Read the model definition and answer for the solid it produces. Units are mm, in the model's axes. Face numbers are marked on the shaded views. A direction names the side the tool comes from. Round coordinates to 2 decimals unless told otherwise and drop trailing zeros. Loops run counter-clockwise (first coordinate to the right, second up) from the corner with the lowest first, then second, coordinate; pieces in that order, holes last. Notation, with made-up numbers: M 57.25,77 L 83.25,77 A23 cw 83.25,105 Z; hole C 42.5,32.25 d1. An arc over 180 degrees is marked long. Write each question's results on one line, items separated by ' | '.
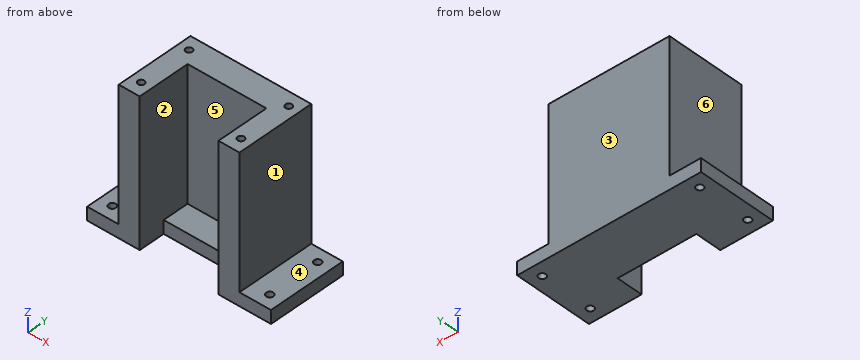
```python
from build123d import *

# Parameters (mm, degrees)
SKETCH_1_R               = 1.35
EXTRUDE_1_DEPTH          = 5
EXTRUDE_2_DEPTH          = 50
SKETCH_3_R               = 1.25
CUT_EXTRUDE_1_DEPTH      = 10
MIRROR_2_COPY_1_SKETCH_R = 1.25
MIRROR_2_COPY_1_DEPTH    = 10


with BuildPart() as part:
    # Sketch 1 → Extrude 1 (new body)
    with BuildSketch(Plane.XY):
        Polygon((20, 0), (20, 10), (50, 10), (50, 0), (70, 0), (70, 30), (0, 30), (0, 0), align=None)
        with Locations((5, 25)):
            Circle(SKETCH_1_R, mode=Mode.SUBTRACT)
        with Locations((5, 5)):
            Circle(SKETCH_1_R, mode=Mode.SUBTRACT)
        with Locations((65, 25)):
            Circle(SKETCH_1_R, mode=Mode.SUBTRACT)
        with Locations((65, 5)):
            Circle(SKETCH_1_R, mode=Mode.SUBTRACT)
    extrude(amount=EXTRUDE_1_DEPTH)

    # Sketch 2 → Extrude 2 (add)
    with BuildSketch(Plane.XY.offset(5)):
        Polygon((20, 20), (20, 0), (12, 0), (12, 30), (58, 30), (58, 0), (50, 0), (50, 20), align=None)
    extrude(amount=EXTRUDE_2_DEPTH)

    # Sketch 3 → Cut-Extrude 1 (cut)
    with BuildSketch(Plane.XY.offset(55)):
        with Locations((16, 25)):
            Circle(SKETCH_3_R)
    cut_extrude_1 = extrude(amount=-CUT_EXTRUDE_1_DEPTH, mode=Mode.SUBTRACT)

    # Mirror 1: Cut-Extrude 1 across plane
    add(cut_extrude_1.mirror(Plane(origin=(35, 0, 0), x_dir=(0, 0, 1), z_dir=(1, 0, 0))), mode=Mode.SUBTRACT)

    # Mirror 2: Cut-Extrude 1 across plane
    add(cut_extrude_1.mirror(Plane.ZX.offset(15)), mode=Mode.SUBTRACT)

    # Mirror 2 copy 1 sketch → Mirror 2 copy 1 (cut)
    with BuildSketch(Plane(origin=(70, 30, 55), x_dir=(-1, 0, 0), z_dir=(0, 0, 1))):
        with Locations((16, 25)):
            Circle(MIRROR_2_COPY_1_SKETCH_R)
    extrude(amount=-MIRROR_2_COPY_1_DEPTH, mode=Mode.SUBTRACT)


solid = part.part
```
1. Which of the six approach directions +Z, -Z, +X, -X, +Y, -Y give full straight-line access (tool end or side, diameter ignored) to the marked faces 4, 5 and 6?
Completed:
face 4: +Z, +X, +Y, -Y | face 5: +Z, -Y | face 6: +Z, -X, +Y, -Y
2. Find the intervals of material crossed by L1, parallel to Y at x = 65, z = 3.85; L2, parallel to X at y = 5, z = 52; L3, parallel to X at y = 11, z = 12, in increasing order.
Completed:
L1: y = 0 to 3.65, 6.35 to 23.65, 26.35 to 30 | L2: x = 12 to 14.75, 17.25 to 20, 50 to 52.75, 55.25 to 58 | L3: x = 12 to 20, 50 to 58
3. Find section B-B, the plane x = 5. Give the vertices of the cut face in (y, z), then the cut area to 3 significant figures.
Completed:
outline: M 0,0 L 3.65,0 L 3.65,5 L 0,5 Z; M 6.35,0 L 23.65,0 L 23.65,5 L 6.35,5 Z; M 26.35,0 L 30,0 L 30,5 L 26.35,5 Z | area: 123 mm2
4. Determine the mould class of the marked faces 1, 2 and 3 for opening direction X: released by +X, released by -X, zero draft, split by the parting line, or undercut.
Completed:
face 1: released by +X | face 2: undercut | face 3: zero draft
5. Find section D-D, the plane y = 2.5. Give the vertices of the cut face in (x, z).
Completed:
outline: M 0,0 L 20,0 L 20,55 L 12,55 L 12,5 L 0,5 Z; M 50,0 L 70,0 L 70,5 L 58,5 L 58,55 L 50,55 Z
6. Find section A-A, the plane y = 25. Give the vertices of the cut face in (x, z), then the cut area to 3 significant figures.
Completed:
outline: M 0,0 L 3.65,0 L 3.65,5 L 0,5 Z; M 6.35,0 L 63.65,0 L 63.65,5 L 58,5 L 58,55 L 55.25,55 L 55.25,45 L 52.75,45 L 52.75,55 L 17.25,55 L 17.25,45 L 14.75,45 L 14.75,55 L 12,55 L 12,5 L 6.35,5 Z; M 66.35,0 L 70,0 L 70,5 L 66.35,5 Z | area: 2,570 mm2
7. Given P1, Ø9, axis at y = 19, z = 42, coming from the -X side; P2, Ø5, axis at x = 25.5, y = 7, coming from the -Z side; P3, Ø5, axis at x = 35, y = 15.5, coming from the +Z side; P4, Ø9, axis at x = 34, z = 33.5, coming from the -Y side, each flat-ended and moving along its own axis, determine where each tip first touches the part or whether it passes through.
Completed:
P1: stops at x = 12 | P2: passes through | P3: stops at z = 5 | P4: stops at y = 20
8. Find section C-C, the plane z = 46. Give the vertices of the cut face in (x, y).
Completed:
outline: M 12,0 L 20,0 L 20,20 L 50,20 L 50,0 L 58,0 L 58,30 L 12,30 Z; hole C 16,5 d2.5; hole C 16,25 d2.5; hole C 54,5 d2.5; hole C 54,25 d2.5
